Autodesk Inventor part; units mm, degrees
ref_plane "YZ Plane" through (0, 0, 0) normal (1, 0, 0) x (0, 1, 0)
ref_plane "XZ Plane" through (0, 0, 0) normal (0, 1, 0) x (-1, 0, 0)
ref_plane "XY Plane" through (0, 0, 0) normal (0, 0, 1) x (1, 0, 0)
sketch "Sketch1" plane through (0, 0, 0) normal (0, 0, 1) x (1, 0, 0)
  line L0 (-51.45, 7.45) -> (40.55, 7.45)
  line L1 (51.45, -5.45) -> (51.45, -7.45)
  line L2 (51.45, -7.45) -> (-51.45, -7.45)
  line L3 (-51.45, -7.45) -> (-51.45, 7.45)
  line L4 (-51.45, 7.45) -> (51.45, -7.45) construction
  line L5 (51.45, 7.45) -> (-51.45, -7.45) construction
  line L6 (40.55, 7.45) -> (40.55, -5.45)
  line L7 (40.55, -5.45) -> (51.45, -5.45)
  point P0 (0, 0)
  dimension "d0" = 102.9
  dimension "d1" = 14.9
  dimension "d2" = 12.9
  dimension "d3" = 10.9
extrude "Extrusion1" add sketch "Sketch1" along normal blind 58.8
sketch "Sketch2" plane through (40.55, -5.45, 0) normal (1, 0, 0) x (0, 0, -1)
  line L0 (0, 0) -> (-58.8, 0)
  line L1 (-58.8, 0) -> (-2, 0)
  line L2 (-2, 0) -> (-2, 2.25)
  line L3 (-2, 2.25) -> (-56.8, 2.25)
  line L4 (-58.8, 2.25) -> (-58.8, 0)
  line L5 (0, 12.9) -> (0, 0)
  line L6 (-56.8, 2.25) -> (-56.8, 0)
  line L7 (-56.8, 4.8) -> (-2, 4.8)
  line L8 (-2, 4.8) -> (-2, 2.55)
  line L9 (-2, 2.55) -> (-56.8, 2.55)
  line L10 (-58.8, 4.8) -> (-2, 2.55) construction
  line L11 (-2, 4.8) -> (-58.8, 2.55) construction
  line L12 (-56.8, 4.8) -> (-56.8, 2.6292)
  line L13 (-56.8, 5.1) -> (-2, 5.1)
  line L14 (-2, 5.1) -> (-2, 7.35)
  line L15 (-2, 7.35) -> (-56.8, 7.35)
  line L16 (-56.8, 7.35) -> (-56.8, 5.1)
  line L17 (-56.8, 5.1) -> (-2, 7.35) construction
  line L18 (-2, 5.1) -> (-56.8, 7.35) construction
  line L19 (-58.8, 0) -> (-58.8, 12.9)
  line L20 (-56.8, 10.9) -> (-2, 10.9)
  line L21 (-2, 10.9) -> (-2, 8.7469)
  line L22 (-2, 8.7469) -> (-56.8, 8.7469)
  line L23 (-56.8, 8.7469) -> (-56.8, 10.9)
  line L24 (-56.8, 10.9) -> (-2, 8.7469) construction
  line L25 (-2, 10.9) -> (-56.8, 8.7469) construction
  line L26 (0, 12.9) -> (-58.8, 12.9)
  point P0 (0, 5.45)
  point P1 (-30.4, 3.675)
  point P2 (-29.4, 6.225)
  point P3 (-29.4, 9.8235)
  dimension "d6" = 56.8
  dimension "d7" = 2.25
  dimension "d8" = 2
  dimension "d9" = 2.25
  dimension "d10" = 2
  dimension "d11" = 0.3
  dimension "d12" = 2.25
  dimension "d13" = 2
  dimension "d14" = 0.3
  dimension "d15" = 2.25
  dimension "d16" = 2
  dimension "d17" = 2
  dimension "d18" = 2
  dimension "d19" = 2
  dimension "d20" = 2.25
properties part number "cardBox_attempt1"
For this review, take the finished solid that the model builds, in its own axes (mm). A direction names the side the tool comes from. Round coordinates to 2 decimals unless told otherwise and drop trailing zeros. Write each loop counter-clockwise with the first axis right and the second up, starting at its lowest first coordinate (ties: lowest second). Pieces come first, ordered by that corner, then holes. Notation, with made-up numbers: M 84.5,2 L 119.5,2 A16 ccw 119.5,28 Z; hole C 87.5,-5.5 d9. An arc over 180 degrees is marked long. One line per item, written item: value. Start each with the question number.
(1) We need section A-A (z = 4). Give the boundary of the cut face in (x, y).
(2) Machinability: for faces 1 (the flat face through (46, -5.45, 29)), 2 (the flat face through (-1, 0, 0)), which of the approach directions +Z, -Z, +X, -X, +Y, -Y give a long, thin tool a straight path to every point of the face, cutting with its end or side? Answer none if there is none.
(3) We need section B-B (y = 4). Give the boundary of the cut face in (x, z), and give its area (3 significant figures).
(4) Insertion check: pin 1 (8 mm diameter, centred on y = 0, z = 42, fed in from +X); pin 2 (3.5 mm diameter, centred on x = 47.5, z = 41, fed in from +Y). Each pin has a flat end and moves straight along its axis. Give the tip position at first contact, or say it passes through.
(5) Wall thickness on line 1 (X direction, y = -3.5, z = 39): over which ranges is the line inside the solid? List them lowest first.
Result:
1. outline: M -51.45,-7.45 L 51.45,-7.45 L 51.45,-5.45 L 40.55,-5.45 L 40.55,7.45 L -51.45,7.45 Z
2. face 1: +Z, -Z, +X, +Y
2. face 2: -Z, +X, -X, +Y, -Y
3. outline: M -51.45,0 L 40.55,0 L 40.55,58.8 L -51.45,58.8 Z
3. area: 5,410 mm²
4. pin 1: x = 40.55
4. pin 2: y = -5.45
5. line 1: -51.45 to 40.55
